Part print with two shaded views. Sizes in mm from the minimum x, y, z corner. A direction names the side the tool comes from. Give positions to 0.01 mm unless a question says otherwise; leave off trailing zeros. Order: outer loops, then holes, each group sorted by start corner. A loop starts at its lowest first (then second) coordinate and runs counter-clockwise, first axis right, second up. Notation, with made-up numbers: M 48,31 L 60,31 A16 ccw 60,47 Z; hole C 38,12.5 d11. An arc over 180 degrees is marked long. Return JSON: item names as keys, results as strings. Group by question number.
1. Slice it at C-C on z = 17. List the corners of the cut face in (x, y).
2. Slice it at A-A on x = 80. List the corners of the cut face in (y, z).
3. Two-plate mould, pull along Z, no slides. Class the marked faces 1, 2 and 3: released by +Z, released by -Z, zero draft, split by the parting line, or undercut.
4. 3-axis set-ups, long thin cutter, end or side, ignore diameter. For the marked faces 4, 5, 6 and 7: which of +Z, -Z, +X, -X, +Y, -Y reach the whole face in a straight line?
5. Slice it at B-B on y = 4. List the corners of the cut face in (x, z), then the cut area to 3 significant figures.
6. Wall check: probe 1 along Y at (x, z) = (80, 55.3); probe 2 along Z at (x, y) = (23.5, 7); probe 3 along Y at (x, z) = (62, 18). Give the ranges that are in metal, low to high. Write a range as [from, to].
7. Pin check, flat tips, straight feed: pin 1 (3 mm diameter, centred on x = 61, z = 29.5, fed in from +Y); pin 2 (6 mm diameter, centred on x = 31.5, y = 6, fed in from +Z); pin 3 (5.5 mm diameter, centred on x = 15, y = 6.5, fed in from -Z). Stop position of each tip, or through.
8. Slice it at D-D on x = 7. List the corners of the cut face in (y, z), then the cut area to 3 significant figures.
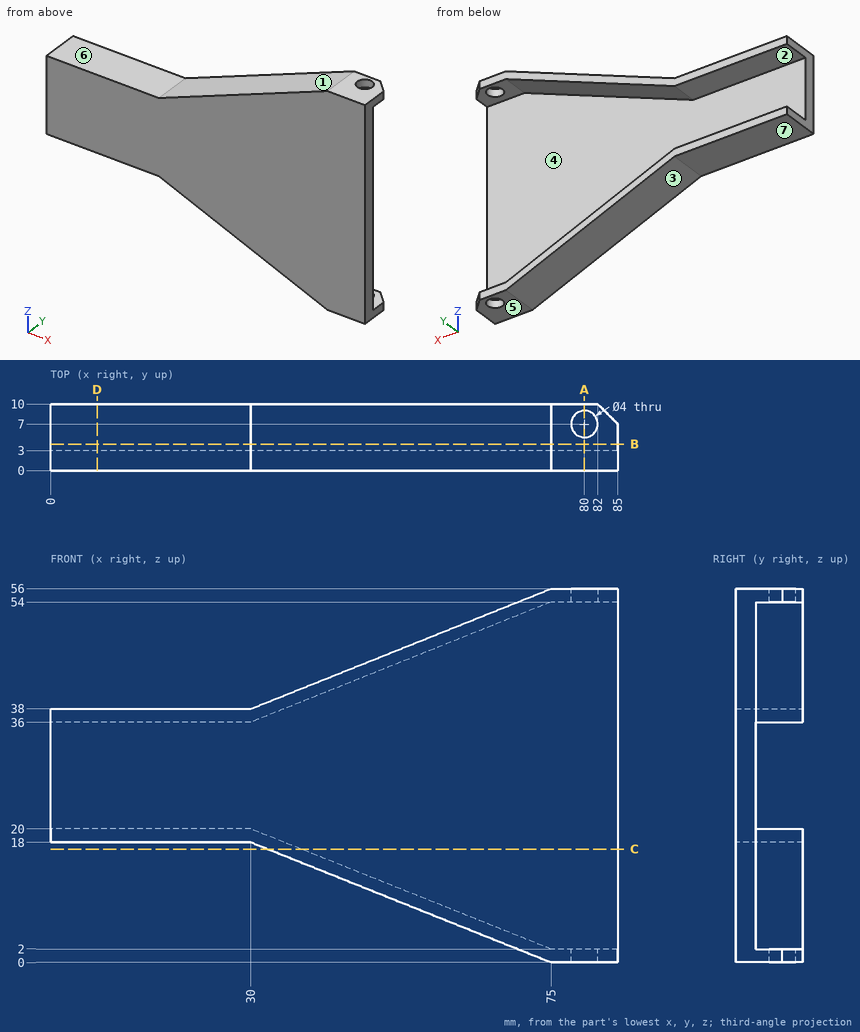
Result:
{
 "1": {"outline": "M 32.5,0 L 85,0 L 85,3 L 37.5,3 L 37.5,10 L 32.5,10 Z"},
 "2": {"outline": "M 0,0 L 5,0 L 5,2 L 3,2 L 3,54 L 5,54 L 5,56 L 0,56 Z; M 9,0 L 10,0 L 10,2 L 9,2 Z; M 9,54 L 10,54 L 10,56 L 9,56 Z"},
 "3": {"face 1": "released by +Z", "face 2": "undercut", "face 3": "released by -Z"},
 "4": {"face 4": "+X, +Y", "face 5": "-Z, +X, -X, +Y, -Y", "face 6": "+Z, -X, +Y, -Y", "face 7": "-Z, -X, +Y, -Y"},
 "5": {"outline": "M 0,18 L 30,18 L 75,0 L 85,0 L 85,2 L 75,2 L 30,20 L 0,20 Z; M 0,36 L 30,36 L 75,54 L 85,54 L 85,56 L 75,56 L 30,38 L 0,38 Z", "area": "340 mm2"},
 "6": {"probe 1": "y = [0, 5], [9, 10]", "probe 2": "z = [18, 20], [36, 38]", "probe 3": "y = [0, 3]"},
 "7": {"pin 1": "stops at y = 3", "pin 2": "stops at z = 39.8", "pin 3": "stops at z = 18"},
 "8": {"outline": "M 0,18 L 10,18 L 10,20 L 3,20 L 3,36 L 10,36 L 10,38 L 0,38 Z", "area": "88.0 mm2"}
}
